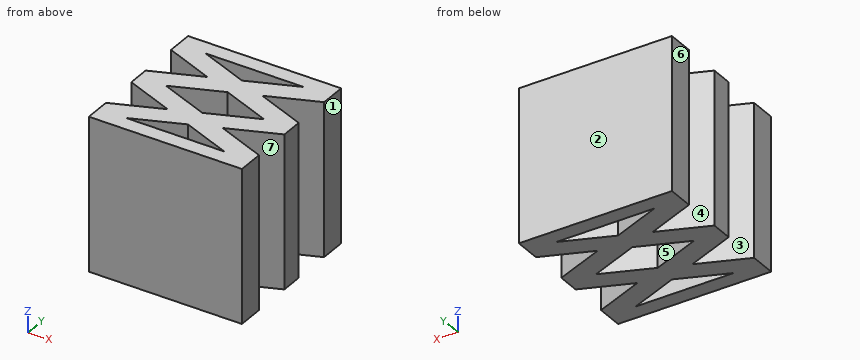
Autodesk Inventor part; units mm, degrees
ref_plane "YZ Plane" through (0, 0, 0) normal (1, 0, 0) x (0, 1, 0)
ref_plane "XZ Plane" through (0, 0, 0) normal (0, 1, 0) x (-1, 0, 0)
ref_plane "XY Plane" through (0, 0, 0) normal (0, 0, 1) x (1, 0, 0)
sketch "Sketch1" plane through (0, 0, 0) normal (0, 0, 1) x (1, 0, 0)
  line L0 (0, 0) -> (30, 0) construction
  line L1 (30, 0) -> (30, 30) construction
  line L2 (30, 30) -> (0, 30) construction
  line L3 (0, 30) -> (0, 0) construction
  line L4 (0, 0) -> (30, 0)
  line L5 (36.8144, 0) -> (36.8144, 3)
  line L6 (0, 3) -> (0, 0)
  line L7 (0, 30) -> (30, 30)
  line L8 (30, 30) -> (30, 27)
  line L9 (24.6148, 27) -> (5.3852, 27)
  line L10 (0, 27) -> (0, 30)
  line L11 (0, 15) -> (30, 15) construction
  line L12 (30, 27) -> (0, 15) construction
  line L13 (12.3074, 22.077) -> (30, 15) construction
  line L14 (30, 27) -> (30, 3)
  line L15 (0, 27) -> (0, 3)
  line L16 (24.6148, 27) -> (15, 23.1541)
  line L17 (9.6148, 21) -> (0, 17.1541)
  line L18 (30, 24.8459) -> (20.3852, 21)
  line L19 (5.3852, 27) -> (15, 23.1541)
  line L20 (20.3852, 21) -> (30, 17.1541)
  line L21 (0, 24.8459) -> (9.6148, 21)
  line L22 (20.3852, 9) -> (30, 5.1541)
  line L23 (0, 12.8459) -> (9.6148, 9)
  line L24 (15, 6.8459) -> (24.6148, 3)
  line L25 (24.6148, 15) -> (15, 11.1541)
  line L26 (9.6148, 9) -> (0, 5.1541)
  line L27 (0, 15) -> (15, 9) construction
  line L28 (17.6926, 7.923) -> (30, 3) construction
  line L29 (15, 18.8459) -> (5.3852, 15)
  line L30 (5.3852, 15) -> (15, 11.1541)
  line L31 (36.8144, 3) -> (35.3852, 3)
  line L32 (24.6148, 3) -> (5.3852, 3)
  line L33 (30, 0) -> (30, 3)
  line L34 (30, 15) -> (27.3074, 13.923) construction
  line L35 (15, 9) -> (0, 3) construction
  line L36 (15, 18.8459) -> (24.6148, 15)
  line L37 (30, 12.8459) -> (20.3852, 9)
  line L38 (17.6926, 7.923) -> (5.3852, 3)
  line L39 (0, 9) -> (0, 37.598)
  line L40 (0, 24.8459) -> (0, 17.1541)
  dimension "d0" = 30
  dimension "d1" = 30
  dimension "d2" = 3
  dimension "d3" = 3
extrude "Extrusion1" add sketch "Sketch1" along normal blind 30 contours L6 L15 L26 L23 L17 L21 L10 L7 L8 L14 L18 L20 L37 L22 L33 L4
properties part number "Jack"
Input: part model. Units: mm. Frame: model coordinates. Face numbers are marked on the shaded views. A direction names the side the tool comes from. Coordinates: 2 decimals unless noted, no trailing zeros. Loops run counter-clockwise (first coordinate to the right, second up) from the corner with the lowest first, then second, coordinate; pieces in that order, holes last. Notation, with made-up numbers: M 41.5,45.5 L 91.5,45.5 A13 ccw 91.5,50.5 Z; hole C -22.5,67.5 d11. An arc over 180 degrees is marked long. Use a Markdown table: item, result. Add a question column.
1) Pin query (flat end, axial travel): P1, Ø15.5, axis at x = 10.5, z = 18.5, coming from the -Y side. Return the tip coordinate at first contact, or that it passes through.
2) Section B-B, the plane x = 15.5. Return the cut outline in (y, z), plus the area to 3 significant figures.
3) Section C-C, the plane y = 15.75. Return the cut outline in (x, z).
4) Line query: L1, parallel to Y at x = 23.5, z = 9; L2, parallel to Y at x = 18, z = 16.25; L3, parallel to Y at x = 15.5, z = 26. Output: solid intervals per line, ascending. Write a range as from..to.
5) Section A-A, the plane z = 22.25. Return the cut outline in (x, y), plus the area to 3 significant figures.
6) Draft query along Y for the marked faces 1, 2, 3 and 4. Return one class per face: +Y half, -Y half, draft (parallel to the pull), parting line (faces both ways), or undercut.
7) Section D-D, the plane x = 3. Return the cut outline in (y, z).
8) Set-up query: the marked faces 5, 6 and 7. Return all of +Z, -Z, +X, -X, +Y, -Y with unobstructed straight access to the full face (end or side cutting, diameter ignored); none if empty.
Answer below:
| question | item | result |
|---|---|---|
| 1 | P1 | y = 0 |
| 2 | outline | M 0,0 L 3,0 L 3,30 L 0,30 Z; M 6.65,0 L 11.35,0 L 11.35,30 L 6.65,30 Z; M 18.65,0 L 23.35,0 L 23.35,30 L 18.65,30 Z; M 27,0 L 30,0 L 30,30 L 27,30 Z |
| 2 | area | 462 mm2 |
| 3 | outline | M 0,0 L 7.26,0 L 7.26,30 L 0,30 Z; M 22.74,0 L 30,0 L 30,30 L 22.74,30 Z |
| 4 | L1 | 0..3, 3.45..7.75, 10.25..14.55, 15.45..19.75, 22.25..26.55, 27..30 |
| 4 | L2 | 0..3, 5.65..12.35, 17.65..24.35, 27..30 |
| 4 | L3 | 0..3, 6.65..11.35, 18.65..23.35, 27..30 |
| 5 | outline | M 0,0 L 30,0 L 30,5.15 L 20.39,9 L 30,12.85 L 30,17.15 L 20.39,21 L 30,24.85 L 30,30 L 0,30 L 0,24.85 L 9.61,21 L 0,17.15 L 0,12.85 L 9.61,9 L 0,5.15 Z; hole M 5.39,3 L 24.61,3 L 15,6.85 Z; hole M 5.39,15 L 15,11.15 L 24.61,15 L 15,18.85 Z; hole M 5.39,27 L 15,23.15 L 24.61,27 Z |
| 5 | area | 604 mm2 |
| 6 | face 1 | draft |
| 6 | face 2 | +Y half |
| 6 | face 3 | undercut |
| 6 | face 4 | undercut |
| 7 | outline | M 0,0 L 6.35,0 L 6.35,30 L 0,30 Z; M 11.65,0 L 18.35,0 L 18.35,30 L 11.65,30 Z; M 23.65,0 L 30,0 L 30,30 L 23.65,30 Z |
| 8 | face 5 | +Z, -Z |
| 8 | face 6 | +Z, -Z, -X, +Y, -Y |
| 8 | face 7 | +Z, -Z, +X |
